```python
from build123d import *

# Parameters (mm, degrees)
SKETCH1_W           = 27.686
SKETCH1_H           = 22.86
SKETCH1_W_2         = 25.4
SKETCH1_H_2         = 26.924
BOSS_EXTRUDE1_DEPTH = 19.304


with BuildPart() as part:
    # Sketch1 → Boss-Extrude1 (new body)
    with BuildSketch(Plane.XY):
        Rectangle(SKETCH1_W, SKETCH1_H)
        with Locations((0, 24.892)):
            Rectangle(SKETCH1_W_2, SKETCH1_H_2)
    extrude(amount=BOSS_EXTRUDE1_DEPTH)

    # Sketch3 → 1/4 NPT Tapped Hole1 (revolve, cut)
    with BuildSketch(Plane(origin=(13.843, -3.81, 9.652), x_dir=(0, 0, -1), z_dir=(0, 1, 0))):
        Polygon((0, 0), (0, 13.502347279), (5.5626, 10.16), (5.5626, 9.906), (5.943685794, 9.906), (6.2402847, 0), align=None)
    revolve(axis=Axis((20.193, -3.81, 9.652), (-1, 0, 0)), mode=Mode.SUBTRACT)

    # Sketch4 → 1/4 NPT Tapped Hole2 (revolve, cut)
    with BuildSketch(Plane(origin=(-13.843, -3.81, 9.652), x_dir=(0, 0, 1), z_dir=(0, 1, 0))):
        Polygon((0, 0), (0, 13.502347279), (5.5626, 10.16), (5.5626, 9.906), (5.943685794, 9.906), (6.2402847, 0), align=None)
    revolve(axis=Axis((-20.193, -3.81, 9.652), (1, 0, 0)), mode=Mode.SUBTRACT)


solid = part.part
```
Could you check a few things on this model? Use its own coordinates, in mm. A direction names the side the tool comes from. Coordinates: 2 decimals unless noted, no trailing zeros. Order: outer loops, then holes, each group sorted by start corner. A loop starts at its lowest first (then second) coordinate and runs counter-clockwise, first axis right, second up. Notation, with made-up numbers: M 71,65.5 L 77,65.5 A20 ccw 77,104.5 Z; hole C 11.5,-23 d8. An arc over 180 degrees is marked long. Use a Markdown table: item, result. Add a question column.
Q1. We'd pull the mould along Z, two halves only. Please class faces 6 (the flat face through (0, 14, 19.304)), 7 (the flat face through (-12.7, 25, 10)), 8 (the conical face through (-0.92, -3.22, 8.89)), 9 (the flat face through (-3.937, 0, 14)): pulls with the +Z half, pulls with the -Z half, needs draft (parallel to the pull), parting line crosses it, or undercut.
Q2. I'm going to push flat-ended pins straight in: pin 1 (2 mm diameter, centred on y = 17, z = 9.5, fed in from -X); pin 2 (0.6 mm diameter, centred on x = -13.5, z = 12, fed in from +Y); pin 3 (9.5 mm diameter, centred on y = -4.5, z = 9, fed in from -X). Where does each tip first touch, or does it pass through?
Q3. I want a section at B-B on y = 21. List the corners of the cut face in (x, z) for me, then the cut area to 3 significant figures.
Q4. If I drill on L1, parallel to Z at x = -3.75, y = -3.81; L2, parallel to Y at x = -7.25, z = 14.75; L3, parallel to Y at x = 11, z = 4.5, over which ranges is the centre line in solid material (lowest first)?
Q5. Which directions (+Z, -Z, +X, -X, +Y, -Y) give clear straight access to the entire face, cutting with the end or side of a thin tool? Please do faces 1 (the conical face through (-8.959, -1.476, 15.281)), 2 (the flat face through (3.937, 0, 14)), 3 (the flat face through (-13, 11.43, 10)), 4 (the flat face through (13, 11.43, 10)), 5 (the flat face through (13.843, 2.4, 11.7)).
Q6. I want a section at C-C on x = -10.25. List the corners of the cut face in (y, z) for me, then the cut area to 3 significant figures.
Q7. I want a section at A-A on x = 6.75. List the corners of the cut face in (y, z) for me.
Checked values:
| question | item | result |
|---|---|---|
| 1 | face 6 | pulls with the +Z half |
| 1 | face 7 | needs draft |
| 1 | face 8 | undercut |
| 1 | face 9 | undercut |
| 2 | pin 1 | x = -12.7 |
| 2 | pin 2 | y = 11.43 |
| 2 | pin 3 | x = -3.94 |
| 3 | outline | M -12.7,0 L 12.7,0 L 12.7,19.3 L -12.7,19.3 Z |
| 3 | area | 490 mm² |
| 4 | L1 | 0 to 4.09, 15.21 to 19.3 |
| 4 | L2 | -11.43 to -7.05, -0.57 to 38.35 |
| 4 | L3 | -11.43 to -7.18, -0.44 to 38.35 |
| 5 | face 1 | -X |
| 5 | face 2 | +X |
| 5 | face 3 | +Z, -Z, -X, +Y |
| 5 | face 4 | +Z, -Z, +X, +Y |
| 5 | face 5 | +Z, -Z, +X, +Y, -Y |
| 6 | outline | M -11.43,0 L 38.35,0 L 38.35,19.3 L -11.43,19.3 Z; hole C -3.81,9.65 d12.27 |
| 6 | area | 843 mm² |
| 7 | outline | M -11.43,0 L 38.35,0 L 38.35,19.3 L -11.43,19.3 Z; hole C -3.81,9.65 d12.06 |
